Design review of the part built by this model. Coordinates are the model's own, in mm. A direction names the side the tool comes from. Give positions to 0.01 mm unless a question says otherwise; leave off trailing zeros. Loops run counter-clockwise (first coordinate to the right, second up) from the corner with the lowest first, then second, coordinate; pieces in that order, holes last. Notation, with made-up numbers: M -7,27 L 28,27 A20 cw 28,45 Z; hole C 55.5,38 d8. An arc over 180 degrees is marked long. Use CSV: the item, a comma, the result in double quotes.
from build123d import *

# Parameters (mm, degrees)
F0_R     = 10.8121335874
F0_W     = 5.7772109285
F0_H     = 0.716982875
F0_H_2   = 0.7141863704
F0_H_3   = 0.5685804115
F1_DEPTH = 3.175


with BuildPart() as f1:
    # F0 (on Front) → F1 (new body)
    with BuildSketch(Plane.XZ):
        Circle(F0_R)
        with BuildLine():
            ThreePointArc((6.3062577959, 7.1383988129), (8.6831080411, 3.9152598569), (9.525, 0))
            ThreePointArc((9.525, 0), (8.6816518395, -3.9184877615), (6.3009482756, -7.1430858757))
            ThreePointArc((6.3009482756, -7.1430858757), (6.2763830489, -7.1646800922), (6.2517438163, -7.1861898288))
            ThreePointArc((6.2517438163, -7.1861898288), (6.2295179256, -7.205465385), (6.2072326042, -7.2246722))
            ThreePointArc((6.2072326042, -7.2246722), (3.3098808358, -8.9314228347), (0, -9.525))
            ThreePointArc((0, -9.525), (-3.3121824388, -8.9305695503), (-6.2109555135, -7.2214719143))
            ThreePointArc((-6.2109555135, -7.2214719143), (-6.2313746359, -7.2038597395), (-6.2517438163, -7.1861898288))
            ThreePointArc((-6.2517438163, -7.1861898288), (-6.2787205913, -7.1626316907), (-6.305608594, -7.1389722831))
            ThreePointArc((-6.305608594, -7.1389722831), (-8.6829300025, -3.9156546797), (-9.525, 0))
            ThreePointArc((-9.525, 0), (-8.7048463851, 3.8666877831), (-6.3856247955, 7.0674904295))
            ThreePointArc((-6.3856247955, 7.0674904295), (-6.3189630276, 7.1271544992), (-6.2517438163, 7.1861898288))
            ThreePointArc((-6.2517438163, 7.1861898288), (-6.1734679548, 7.2535452305), (-6.0944664659, 7.3200480529))
            ThreePointArc((-6.0944664659, 7.3200480529), (-3.2405375554, 8.9568153577), (0, 9.525))
            ThreePointArc((0, 9.525), (3.2811323241, 8.9420241373), (6.1606224546, 7.2644584087))
            ThreePointArc((6.1606224546, 7.2644584087), (6.2063065187, 7.2254677632), (6.2517438163, 7.1861898288))
            ThreePointArc((6.2517438163, 7.1861898288), (6.2790462746, 7.1623461855), (6.3062577959, 7.1383988129))
        make_face(mode=Mode.SUBTRACT)
        with Locations((-2.8886054642, 4.8158199061)):
            Rectangle(F0_W, F0_H)
        with Locations((2.8886054642, 4.8158199061)):
            Rectangle(F0_W, F0_H)
        with Locations((-2.8886054642, 0.5223121699)):
            Rectangle(F0_W, F0_H)
        with Locations((2.8886054642, 0.5223121699)):
            Rectangle(F0_W, F0_H)
        with Locations((2.8886054642, -3.7711955662)):
            Rectangle(F0_W, F0_H)
        with Locations((-2.8886054642, -3.7711955662)):
            Rectangle(F0_W, F0_H)
        with Locations((-2.8886054642, 2.669066038)):
            Rectangle(F0_W, F0_H_2)
        with Locations((2.8886054642, 2.669066038)):
            Rectangle(F0_W, F0_H_2)
        with Locations((-2.8886054642, -1.6244416981)):
            Rectangle(F0_W, F0_H_2)
        with Locations((2.8886054642, -1.6244416981)):
            Rectangle(F0_W, F0_H_2)
        Polygon((5.7772109285, 6.605480589), (6.2517438163, 7.1861898288), (6.0889851302, 7.1861898288), (0, 7.1861898288), (0, 6.605480589), align=None)
        Polygon((0, 6.605480589), (0, 7.1861898288), (-5.9895003214, 7.1861898288), (-6.2517438163, 7.1861898288), (-5.7772109285, 6.605480589), align=None)
        Polygon((-6.1821243726, -7.1861898288), (0, -7.1861898288), (0, -6.605480589), (-5.7772109285, -6.605480589), (-6.2517438163, -7.1861898288), align=None)
        Polygon((6.1562946066, -7.1861898288), (6.2517438163, -7.1861898288), (5.7772109285, -6.605480589), (0, -6.605480589), (0, -7.1861898288), align=None)
        with Locations((-2.8886054642, -5.8451464548)):
            Rectangle(F0_W, F0_H_3)
        with Locations((2.8886054642, -5.8451464548)):
            Rectangle(F0_W, F0_H_3)
        Polygon((6.2517438163, -7.1099842899), (6.2517438163, 0), (5.7772109285, 0), (5.7772109285, -0.5503656379), (5.7772109285, -1.2673485129), (5.7772109285, -1.9815348833), (5.7772109285, -2.6985177583), (5.7772109285, -3.4127041287), (5.7772109285, -4.1296870037), (5.7772109285, -4.843873374), (5.7772109285, -5.5608562491), (5.7772109285, -6.1294366606), (5.7772109285, -6.605480589), (6.2517438163, -7.1861898288), align=None)
        Polygon((5.7772109285, 0), (6.2517438163, 0), (6.2517438163, 7.0716873743), (6.2517438163, 7.1861898288), (5.7772109285, 6.605480589), (5.7772109285, 5.8884977139), (5.7772109285, 5.1743113436), (5.7772109285, 4.4573284686), (5.7772109285, 3.7431420982), (5.7772109285, 3.0261592232), (5.7772109285, 2.3119728528), (5.7772109285, 1.5949899778), (5.7772109285, 0.8808036075), (5.7772109285, 0.1638207324), align=None)
        Polygon((-6.2517438163, 0), (-5.7772109285, 0), (-5.7772109285, 0.1638207324), (-5.7772109285, 0.8808036075), (-5.7772109285, 1.5949899778), (-5.7772109285, 2.3119728528), (-5.7772109285, 3.0261592232), (-5.7772109285, 3.7431420982), (-5.7772109285, 4.4573284686), (-5.7772109285, 5.1743113436), (-5.7772109285, 5.8884977139), (-5.7772109285, 6.605480589), (-6.2517438163, 7.1861898288), (-6.2517438163, 6.9398786873), align=None)
        Polygon((-5.7772109285, -0.5503656379), (-5.7772109285, 0), (-6.2517438163, 0), (-6.2517438163, -7.1003455669), (-6.2517438163, -7.1861898288), (-5.7772109285, -6.605480589), (-5.7772109285, -6.1294366606), (-5.7772109285, -5.5608562491), (-5.7772109285, -4.843873374), (-5.7772109285, -4.1296870037), (-5.7772109285, -3.4127041287), (-5.7772109285, -2.6985177583), (-5.7772109285, -1.9815348833), (-5.7772109285, -1.2673485129), align=None)
        with BuildLine():
            Line((-5.9895003214, 7.1861898288), (-6.0944664659, 7.3200480529))
            ThreePointArc((-6.0944664659, 7.3200480529), (-6.1734679548, 7.2535452305), (-6.2517438163, 7.1861898288))
            Line((-6.2517438163, 7.1861898288), (-5.9895003214, 7.1861898288))
        make_face()
        with BuildLine():
            Line((-6.2517438163, 6.9398786873), (-6.2517438163, 7.1861898288))
            ThreePointArc((-6.2517438163, 7.1861898288), (-6.3189630276, 7.1271544992), (-6.3856247955, 7.0674904295))
            Line((-6.3856247955, 7.0674904295), (-6.2517438163, 6.9398786873))
        make_face()
        with BuildLine():
            Line((6.0889851302, 7.1861898288), (6.2517438163, 7.1861898288))
            ThreePointArc((6.2517438163, 7.1861898288), (6.2063065187, 7.2254677632), (6.1606224546, 7.2644584087))
            Line((6.1606224546, 7.2644584087), (6.0889851302, 7.1861898288))
        make_face()
        with BuildLine():
            Line((6.2517438163, 7.0716873743), (6.3062577959, 7.1383988129))
            ThreePointArc((6.3062577959, 7.1383988129), (6.2790462746, 7.1623461855), (6.2517438163, 7.1861898288))
            Line((6.2517438163, 7.1861898288), (6.2517438163, 7.0716873743))
        make_face()
        with BuildLine():
            ThreePointArc((-6.305608594, -7.1389722831), (-6.2787205913, -7.1626316907), (-6.2517438163, -7.1861898288))
            Line((-6.2517438163, -7.1861898288), (-6.2517438163, -7.1003455669))
            Line((-6.2517438163, -7.1003455669), (-6.305608594, -7.1389722831))
        make_face()
        with BuildLine():
            ThreePointArc((6.2517438163, -7.1861898288), (6.2763830489, -7.1646800922), (6.3009482756, -7.1430858757))
            Line((6.3009482756, -7.1430858757), (6.2517438163, -7.1099842899))
            Line((6.2517438163, -7.1099842899), (6.2517438163, -7.1861898288))
        make_face()
        with BuildLine():
            ThreePointArc((6.2072326042, -7.2246722), (6.2295179256, -7.205465385), (6.2517438163, -7.1861898288))
            Line((6.2517438163, -7.1861898288), (6.1562946066, -7.1861898288))
            Line((6.1562946066, -7.1861898288), (6.2072326042, -7.2246722))
        make_face()
        with BuildLine():
            ThreePointArc((-6.2517438163, -7.1861898288), (-6.2313746359, -7.2038597395), (-6.2109555135, -7.2214719143))
            Line((-6.2109555135, -7.2214719143), (-6.1821243726, -7.1861898288))
            Line((-6.1821243726, -7.1861898288), (-6.2517438163, -7.1861898288))
        make_face()
    extrude(amount=F1_DEPTH)


solid = f1.part
(1) Clearance check with flat-ended pins moving along their axes: P1, Ø1, axis at x = 7, y = -0.5, coming from the +Z side; P2, Ø1.1, axis at y = -2, z = 1.5, coming from the -X side; P3, Ø1.5, axis at x = 1, y = -2.5, coming from the -Z side. State where each tip first meets the part, or that it passes through.
A:
P1,"z = 8.64"
P2,"x = -10.77"
P3,"z = -10.81"
(2) Wall thickness on line 1 along X through (y, z) = (-1.5, -5); line 2 along X through (y, z) = (-0.75, 5); line 3 along X through (y, z) = (-2.8, 0.75): over which ranges is each line inside the solid? List them lowest first. Write a range as [from, to].
A:
line 1,"[-9.59, -8.11], [-6.25, -5.78], [5.78, 6.25], [8.11, 9.59]"
line 2,"[-9.59, -8.11], [-6.25, 6.25], [8.11, 9.59]"
line 3,"[-10.79, -9.5], [-6.25, 6.25], [9.5, 10.79]"
(3) We need section C-C on z = 8.25. State the section outline as (x, y) points (3 decimals), then the cut area to 3 significant figures.
A:
outline,"M -6.989,-3.175 L -4.761,-3.175 L -4.761,0 L -6.989,0 Z; M 4.761,-3.175 L 6.989,-3.175 L 6.989,0 L 4.761,0 Z"
area,"14.1 mm²"
(4) We need section A-A on z = 2. State the section outline as (x, y) points (3 decimals).
A:
outline,"M -10.626,-3.175 L -9.313,-3.175 L -9.313,0 L -10.626,0 Z; M -6.252,-3.175 L -5.777,-3.175 L -5.777,0 L -6.252,0 Z; M 5.777,-3.175 L 6.252,-3.175 L 6.252,0 L 5.777,0 Z; M 9.313,-3.175 L 10.626,-3.175 L 10.626,0 L 9.313,0 Z"
(5) We need section D-D on y = -2. Count the separate pieces of the cut face and the enclosed holes in it, then the cut area to 3 significant figures.
A:
separate pieces,"1"
enclosed holes,"11"
area,"157 mm²"
(6) We need section B-B on x = 7.5. State the section outline as (y, z) points (3 decimals).
A:
outline,"M -3.175,-7.788 L 0,-7.788 L 0,-5.872 L -3.175,-5.872 Z; M -3.175,5.872 L 0,5.872 L 0,7.788 L -3.175,7.788 Z"
(7) The part is to be moulded in two halves that separate along Z. For faces 3 (the flat face through (0, -2, 2.312)), 4 (the flat face through (-0.2, -3.175, 2.6)), say which applies: released by +Z, released by -Z, zero draft, split by the parting line, or undercut.
A:
face 3,"undercut"
face 4,"zero draft"
(8) Machinability: for faces 1 (the flat face through (0, -2, -1.982)), 2 (the flat face through (-0.2, 0, 2.6)), which of the approach directions +Z, -Z, +X, -X, +Y, -Y give a long, thin tool a straight path to every point of the face, cutting with its end or side? Answer none if there is none.
A:
face 1,"+Y, -Y"
face 2,"+Z, -Z, +X, -X, +Y"
